Autodesk Inventor part; units mm, degrees
ref_plane "YZ Plane" through (0, 0, 0) normal (1, 0, 0) x (0, 1, 0)
ref_plane "XZ Plane" through (0, 0, 0) normal (0, 1, 0) x (-1, 0, 0)
ref_plane "XY Plane" through (0, 0, 0) normal (0, 0, 1) x (1, 0, 0)
sketch "Sketch1" plane through (0, 0, 0) normal (0, 1, 0) x (-1, 0, 0)
  line L0 (0, 0) -> (50.8, 0)
  line L1 (50.8, 0) -> (50.8, -25.4)
  line L2 (50.8, -25.4) -> (38.1, -50.8)
  line L3 (38.1, -50.8) -> (12.7, -50.8)
  line L4 (12.7, -50.8) -> (0, -25.4)
  line L5 (0, -25.4) -> (0, 0)
  circle A0 centre (12.7, -12.7) radius 3.175
  circle A1 centre (38.1, -12.7) radius 3.175
  circle A2 centre (25.4, -38.1) radius 3.175
  dimension "d0" = 25.4
  dimension "d1" = 50.8
  dimension "d2" = 25.4
  dimension "d3" = 50.8
  dimension "d4" = 12.7
  dimension "d5" = 6.35
  dimension "d6" = 6.35
  dimension "d7" = 12.7
  dimension "d8" = 12.7
  dimension "d9" = 12.7
  dimension "d10" = 12.7
  dimension "d11" = 6.35
  dimension "d12" = 12.7
  dimension "d13" = 12.7
extrude "Extrusion1" add sketch "Sketch1" along normal blind 3.175
properties part number "15102898-16-P-0212" material "Aluminum 6061"
Build history of the part. All positions in model axes, mm. Give positions to 0.01 mm unless a question says otherwise; leave off trailing zeros. Loops run counter-clockwise (first coordinate to the right, second up) from the corner with the lowest first, then second, coordinate; pieces in that order, holes last. Notation, with made-up numbers: (-19, 47) - (17, 47) arc R14 ccw to (17, 70) - close; hole circle Ø10 at (3, 84). An arc over 180 degrees is marked (long way). Write item = value, one per line. Start each with the question number.
1) Drop flat-ended pins along their axis: pin 1 Ø1.5 at (x, y) = (-40.5, 0.5) entering from -Z; pin 2 Ø1 at (y, z) = (1.5, -40) entering from -X. Give the stop position or say it passes through.
2) Probe probe 1 along Z at (x, y) = (-25.4, 1.55) (3 decimals); probe 2 along X at (y, z) = (2.7, -40.5); probe 3 along Z at (x, y) = (-39, 1.55). List the from-to ranges inside material, lowest first. Write a range as from..to.
3) Pull direction X, two halves, no side cores. Call faces 1 (the flat face through (-25, 0, -25)), 2 (the flat face through (0, 2, -13)), 3 (the cylindrical face through (-10.18, 1.57, -10.77)): +X half, -X half, draft (parallel to the pull), parting line (faces both ways), or undercut.
4) Band-saw the part on B-B on y = 1.65. Give the cut face in (x, z) (3 decimals), plus the area to 3 significant figures.
5) Band-saw the part on D-D on z = -38.1. Give the cut face in (x, y) (3 decimals).
6) Band-saw the part on A-A on x = -25.4. Give the cut face in (y, z) (3 decimals).
7) Band-saw the part on C-C on z = -12.7. Give the cut face in (x, y) (3 decimals), plus the area to 3 significant figures.
Final values:
q1.pin_1 = -47.5
q1.pin_2 = -43.75
q2.probe_1 = -50.8..-41.275, -34.925..0
q2.probe_2 = -43.25..-27.48, -23.32..-7.55
q2.probe_3 = -49..-15.74, -9.66..0
q3.face_1 = draft
q3.face_2 = +X half
q3.face_3 = undercut
q4.outline = (-50.8, -25.4) - (-38.1, -50.8) - (-12.7, -50.8) - (0, -25.4) - (0, 0) - (-50.8, 0) - close; hole circle Ø6.35 at (-38.1, -12.7); hole circle Ø6.35 at (-25.4, -38.1); hole circle Ø6.35 at (-12.7, -12.7)
q4.area = 2,160 mm²
q5.outline = (-44.45, 0) - (-28.575, 0) - (-28.575, 3.175) - (-44.45, 3.175) - close; (-22.225, 0) - (-6.35, 0) - (-6.35, 3.175) - (-22.225, 3.175) - close
q6.outline = (0, -50.8) - (3.175, -50.8) - (3.175, -41.275) - (0, -41.275) - close; (0, -34.925) - (3.175, -34.925) - (3.175, 0) - (0, 0) - close
q7.outline = (-50.8, 0) - (-41.275, 0) - (-41.275, 3.175) - (-50.8, 3.175) - close; (-34.925, 0) - (-15.875, 0) - (-15.875, 3.175) - (-34.925, 3.175) - close; (-9.525, 0) - (0, 0) - (0, 3.175) - (-9.525, 3.175) - close
q7.area = 121 mm²
